Part model, mm, in its own coordinate system. Round coordinates to 2 decimals unless told otherwise and drop trailing zeros. Loops run counter-clockwise (first coordinate to the right, second up) from the corner with the lowest first, then second, coordinate; pieces in that order, holes last. Notation, with made-up numbers: M -36.5,12.25 L -2.5,12.25 A20 ccw -2.5,35.25 Z; hole C -4,13 d4. An arc over 180 degrees is marked long. Put each result on its own line as item: value. Start each with the question number.
1) Slice it at C-C on z = -8. Give the cut face in (x, y).
2) Slice it at A-A on x = 0. Give the cut face in (y, z), then the cut area to 3 significant figures.
3) Probe line 1 along Z through (x, y) = (0, -3.45); line 2 along X through (y, z) = (-3.2, -29); line 3 along X through (y, z) = (-2.4, 16). List the from-to ranges inside material, lowest first.
4) Slice it at B-B on y = -2.3. Give the cut face in (x, z) (1 decimal), then the cut area to 3 significant figures.
5) Slice it at D-D on x = -6.5. Give the cut face in (y, z), then the cut area to 3 significant figures.
```python
from build123d import *

# Parameters (mm, degrees)
BOSS_EXTRUDE1_START = 1
SKETCH1_R           = 25.4
SKETCH1_R_2         = 1
BOSS_EXTRUDE1_DEPTH = 3.175
FILLET1_R           = 4.7625


with BuildPart() as part:
    # Sketch1 → Boss-Extrude1 (new body)
    with BuildSketch(Plane.XZ.offset(0.396875).offset(BOSS_EXTRUDE1_START)):
        Circle(SKETCH1_R)
        with BuildLine():
            Line((4, 29.4), (4, -29.4))
            ThreePointArc((4, -29.4), (0, -33.4), (-4, -29.4))
            Line((-4, -29.4), (-4, 29.4))
            ThreePointArc((-4, 29.4), (0, 33.4), (4, 29.4))
        make_face()
        with Locations((0, 29.4)):
            Circle(SKETCH1_R_2, mode=Mode.SUBTRACT)
        with Locations((0, -29.4)):
            Circle(SKETCH1_R_2, mode=Mode.SUBTRACT)
    extrude(amount=BOSS_EXTRUDE1_DEPTH)

    # Fillet1
    fillet1_edges = [part.edges().sort_by_distance(p)[0] for p in [
        (-4, -2.984375, -25.083062014),
        (-4, -2.984375, 25.083062014),
        (4, -2.984375, 25.083062014),
        (4, -2.984375, -25.083062014),
    ]]
    fillet(fillet1_edges, radius=FILLET1_R)


solid = part.part
```
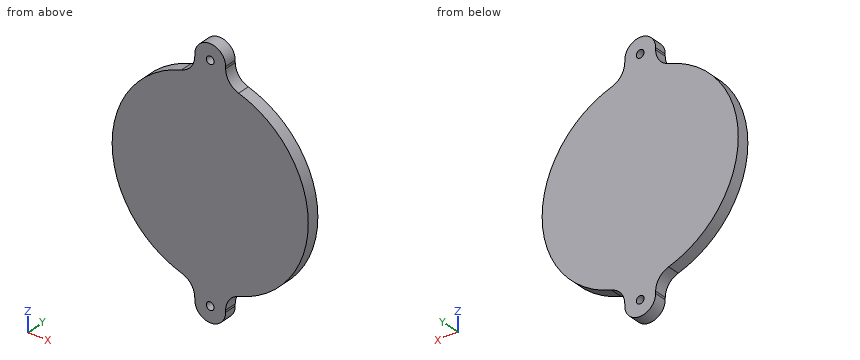
Recorded:
1. outline: M -24.11,-4.57 L 24.11,-4.57 L 24.11,-1.4 L -24.11,-1.4 Z
2. outline: M -4.57,-33.4 L -1.4,-33.4 L -1.4,-30.4 L -4.57,-30.4 Z; M -4.57,-28.4 L -1.4,-28.4 L -1.4,28.4 L -4.57,28.4 Z; M -4.57,30.4 L -1.4,30.4 L -1.4,33.4 L -4.57,33.4 Z
2. area: 199 mm2
3. line 1: z = -33.4 to -30.4, -28.4 to 28.4, 30.4 to 33.4
3. line 2: x = -4 to -0.92, 0.92 to 4
3. line 3: x = -19.73 to 19.73
4. outline: M -7.4,-24.3 A4.8 cw -4,-28.9 L -4,-29.4 A4 ccw 4,-29.4 L 4,-28.9 A4.8 cw 7.4,-24.3 A25.4 ccw 7.4,24.3 A4.8 cw 4,28.9 L 4,29.4 A4 ccw -4,29.4 L -4,28.9 A4.8 cw -7.4,24.3 A25.4 ccw Z; hole C 0,-29.4 d2; hole C 0,29.4 d2
4. area: 2,150 mm2
5. outline: M -4.57,-24.67 L -1.4,-24.67 L -1.4,24.67 L -4.57,24.67 Z
5. area: 157 mm2
